The figure shows three views and two pictorial views of one solid part (mm, origin at its lowest corner). Answer the questions. Coordinates: 2 decimals unless noted, no trailing zeros. Order: outer loops, then holes, each group sorted by start corner. A loop starts at its lowest first (then second) coordinate and runs counter-clockwise, first axis right, second up.
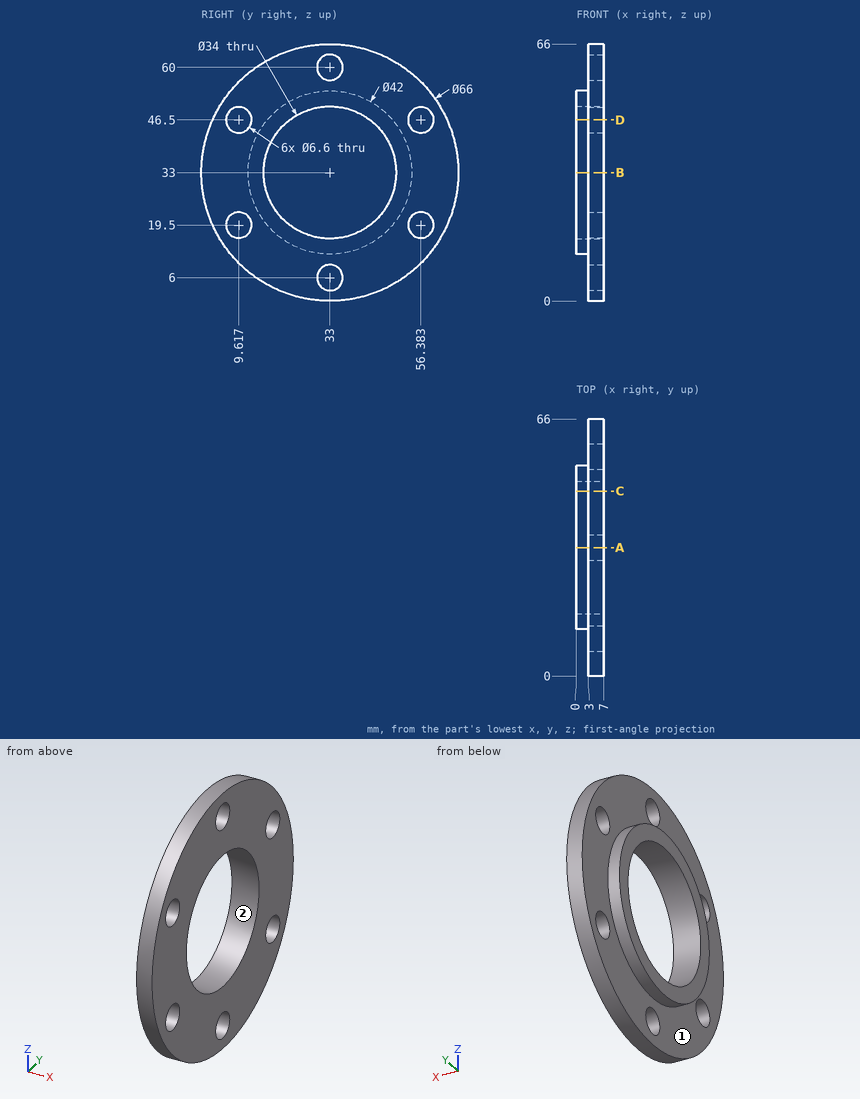
1) A cutting plane is placed at B-B, the plane z = 33. Write down the section's boundary in (x, y), plus the area to 3 significant figures.
2) A cutting plane is placed at D-D, the plane z = 46.5. Write down the section's boundary in (x, y).
3) The mould has two halves that part along Z. Classify the marked faces 1 and 2: released by +Z, released by -Z, zero draft, split by the parting line, or undercut.
4) A cutting plane is placed at A-A, the plane y = 33. Write down the section's boundary in (x, z).
5) Straight lines are drawn through the part: probe 1 along Z at (x, y) = (4.35, 33); probe 2 along Y at (x, z) = (6.5, 33); probe 3 along Z at (x, y) = (1.5, 33). For each, find the intervals that lie inside material, in ascending order.
6) A cutting plane is placed at C-C, the plane y = 47.5. Write down the section's boundary in (x, z).
7) Each of these flat-tipped pins is pushed along its axis until it touches: P1, Ø3, axis at x = 6, y = 45.5, coming from the -Z side; P2, Ø1, axis at x = 3.5, y = 49, coming from the -Z side; P3, Ø10.5, axis at y = 33, z = 60, coming from the -X side. Where does it stop, or does it pass through?
Working result:
1. outline: (0, 12) - (3, 12) - (3, 0) - (7, 0) - (7, 16) - (0, 16) - close; (0, 50) - (7, 50) - (7, 66) - (3, 66) - (3, 54) - (0, 54) - close
1. area: 152 mm2
2. outline: (0, 16.91) - (3, 16.91) - (3, 12.92) - (7, 12.92) - (7, 22.67) - (0, 22.67) - close; (0, 43.33) - (7, 43.33) - (7, 53.08) - (3, 53.08) - (3, 49.09) - (0, 49.09) - close; (3, 2.89) - (7, 2.89) - (7, 6.32) - (3, 6.32) - close; (3, 59.68) - (7, 59.68) - (7, 63.11) - (3, 63.11) - close
3. face 1: zero draft
3. face 2: undercut
4. outline: (0, 12) - (3, 12) - (3, 9.3) - (7, 9.3) - (7, 16) - (0, 16) - close; (0, 50) - (7, 50) - (7, 56.7) - (3, 56.7) - (3, 54) - (0, 54) - close; (3, 0) - (7, 0) - (7, 2.7) - (3, 2.7) - close; (3, 63.3) - (7, 63.3) - (7, 66) - (3, 66) - close
5. probe 1: z = 0 to 2.7, 9.3 to 16, 50 to 56.7, 63.3 to 66
5. probe 2: y = 0 to 16, 50 to 66
5. probe 3: z = 12 to 16, 50 to 54
6. outline: (0, 17.81) - (3, 17.81) - (3, 3.36) - (7, 3.36) - (7, 24.13) - (0, 24.13) - close; (0, 41.87) - (7, 41.87) - (7, 62.64) - (3, 62.64) - (3, 48.19) - (0, 48.19) - close
7. P1: stops at z = 1.89
7. P2: stops at z = 3.87
7. P3: stops at x = 3
